Could you check a few things on this model? Use its own coordinates, in mm. Face numbers are marked on the shaded views. A direction names the side the tool comes from. Round coordinates to 2 decimals unless told otherwise and drop trailing zeros. Order: outer loops, then holes, each group sorted by start corner. A loop starts at its lowest first (then second) coordinate and runs counter-clockwise, first axis right, second up. Notation, with made-up numbers: M -17,52.5 L 14,52.5 A14 cw 14,67.5 Z; hole C 59,89 d10. An arc over 180 degrees is marked long. Write each question's results on one line, items separated by ' | '. Start each with the question number.
1. For the marked faces 4 and 5, which set-ups out of +Z, -Z, +X, -X, +Y, -Y let a thin tool reach every point of the face, with its end or its side?
2. Suppose I cut it at D-D on y = 2.5. Write out the boundary of the cut face in (x, z), and give its area (3 significant figures).
3. I'm going to push flat-ended pins straight in: pin 1 (4.5 mm diameter, centred on x = 58.33, y = 10, fed in from -Z); pin 2 (8 mm diameter, centred on y = 7.5, z = 0.5, fed in from +X). Where does each tip first touch, or does it pass through?
4. We'd pull the mould along Z, two halves only. Please class the marked faces 1, 2 and 3: released by +Z, released by -Z, zero draft, split by the parting line, or undercut.
5. Suppose I cut it at B-B on x = 52. Write out the boundary of the cut face in (y, z).
6. Suppose I cut it at A-A on y = 10. Write out the boundary of the cut face in (x, z).
7. Please list where these lines run through material, in increasing order: L1, parallel to Y at x = 5, z = 5.25; L2, parallel to Z at x = 53.5, y = -2.5; L3, parallel to X at y = 11, z = -9.
8. Suppose I cut it at C-C on z = 6. Write out the boundary of the cut face in (x, y), and give its area (3 significant figures).
from build123d import *

# Parameters (mm, degrees)
ESQUISSE2_W             = 63.33
ESQUISSE2_H             = 20
BOSS_EXTRU_1_DEPTH      = 15
CONG_1_R                = 3
ESQUISSE4_W             = 20
ESQUISSE4_H             = 10
ENL_V_MAT_EXTRU_1_DEPTH = 31
ESQUISSE5_R             = 2.5
ENL_V_MAT_EXTRU_2_DEPTH = 21


with BuildPart() as part:
    # Esquisse2 → Boss.-Extru.1 (new body, symmetric)
    with BuildSketch(Plane(origin=(0, 0, 0), x_dir=(1, 0, 0), z_dir=(0, 1, 0))):
        with Locations((31.665, 0)):
            Rectangle(ESQUISSE2_W, ESQUISSE2_H)
    extrude(amount=BOSS_EXTRU_1_DEPTH, both=True)

    # Congé1
    cong_1_edges = [part.edges().sort_by_distance(p)[0] for p in [
        (63.33, 15, 0),
        (0, 15, 0),
        (63.33, -15, 0),
        (0, -15, 0),
    ]]
    fillet(cong_1_edges, radius=CONG_1_R)

    # Esquisse4 → Enlèv. mat.-Extru.1 (cut, through all)
    with BuildSketch(Plane(origin=(0, 15, 0), x_dir=(1, 0, 0), z_dir=(0, 1, 0))):
        with Locations((53.33, 0)):
            Rectangle(ESQUISSE4_W, ESQUISSE4_H)
    extrude(amount=-ENL_V_MAT_EXTRU_1_DEPTH, mode=Mode.SUBTRACT)

    # Esquisse5 → Enlèv. mat.-Extru.2 (cut, through all)
    with BuildSketch(Plane(origin=(0, 0, -10), x_dir=(-1, 0, 0), z_dir=(0, 0, -1))):
        with Locations((-58.33, 10)):
            Circle(ESQUISSE5_R)
        with Locations((-5, 10)):
            Circle(ESQUISSE5_R)
    extrude(amount=-ENL_V_MAT_EXTRU_2_DEPTH, mode=Mode.SUBTRACT)


solid = part.part
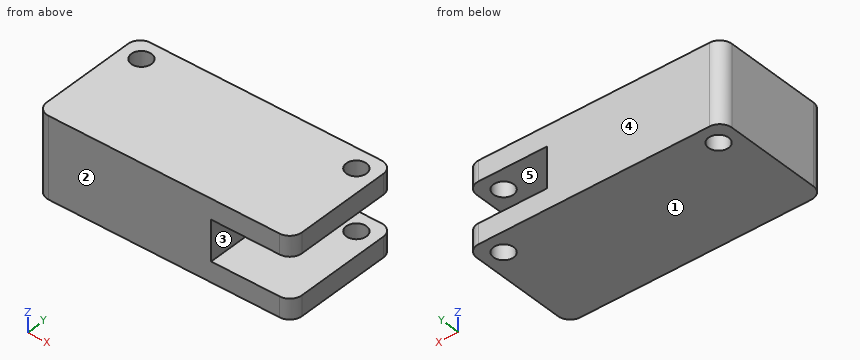
Filled sheet:
1) face 4: +Z, -Z, +X, -X, +Y | face 5: +X, +Y, -Y
2) outline: M 0,-10 L 63.33,-10 L 63.33,-5 L 43.33,-5 L 43.33,5 L 63.33,5 L 63.33,10 L 0,10 Z | area: 1,070 mm^2
3) pin 1: passes through | pin 2: stops at x = 43.33
4) face 1: released by -Z | face 2: zero draft | face 3: undercut
5) outline: M -15,-10 L 15,-10 L 15,-5 L -15,-5 Z; M -15,5 L 15,5 L 15,10 L -15,10 Z
6) outline: M 0,-10 L 2.5,-10 L 2.5,10 L 0,10 Z; M 7.5,-10 L 55.83,-10 L 55.83,-5 L 43.33,-5 L 43.33,5 L 55.83,5 L 55.83,10 L 7.5,10 Z; M 60.83,-10 L 63.33,-10 L 63.33,-5 L 60.83,-5 Z; M 60.83,5 L 63.33,5 L 63.33,10 L 60.83,10 Z
7) L1: y = -15 to 7.5, 12.5 to 15 | L2: z = -10 to -5, 5 to 10 | L3: x = 0 to 2.71, 7.29 to 56.04, 60.62 to 63.33
8) outline: M 0,-12 A3 ccw 3,-15 L 60.33,-15 A3 ccw 63.33,-12 L 63.33,12 A3 ccw 60.33,15 L 3,15 A3 ccw 0,12 Z; hole C 5,10 d5; hole C 58.33,10 d5 | area: 1,850 mm^2
